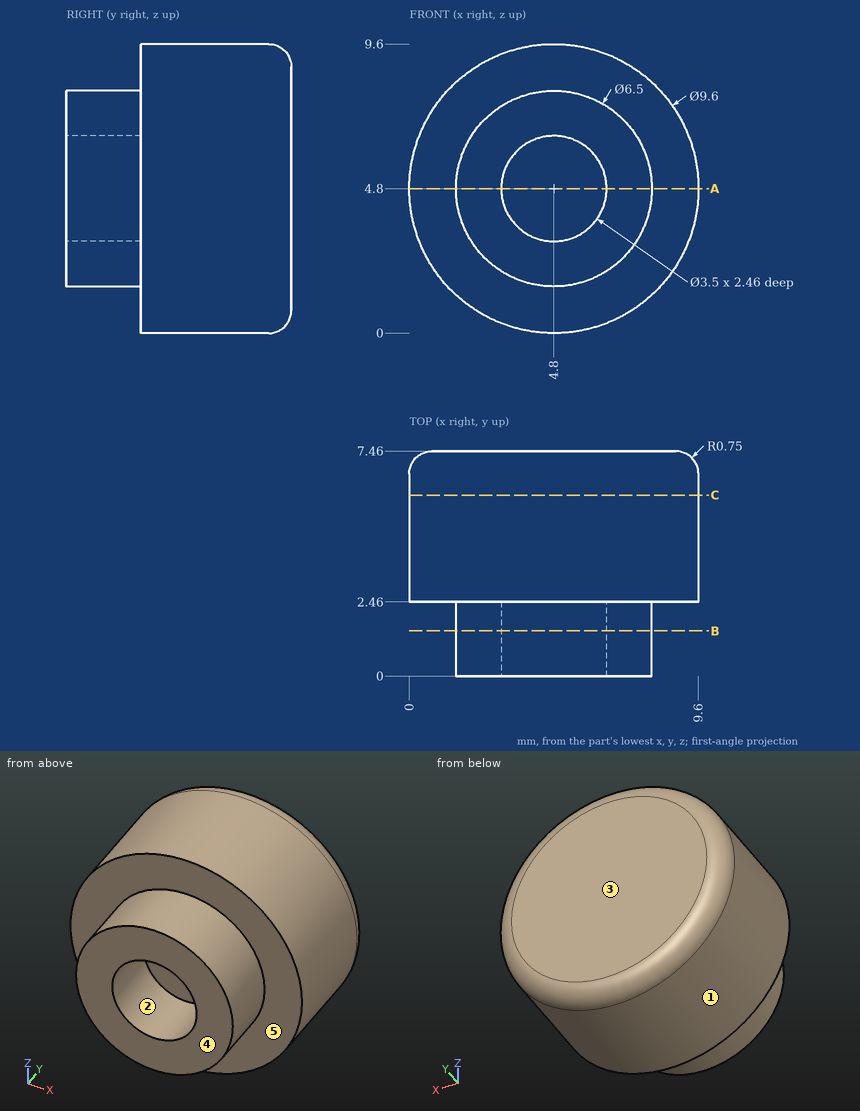
Geometry: see drawing. Coordinates: mm, zero at the bounding-box minimum. A direction names the side the tool comes from. Coordinates: 2 decimals unless noted, no trailing zeros. Loops run counter-clockwise (first coordinate to the right, second up) from the corner with the lowest first, then second, coordinate; pieces in that order, holes last.
(1) Section C-C on y = 6. Return the cut outline in (x, z).
(2) Section A-A on z = 4.8. Return the cut outline in (x, y).
(3) Material intervals for probe 1 along Z at (x, y) = (4.8, 1.4); probe 2 along Y at (x, z) = (1.5, 6.75); probe 3 along X at (y, z) = (1.25, 6.25), sorted ascending.
(4) Set-up query: the marked faces 4 and 5. Return all of +Z, -Z, +X, -X, +Y, -Y with unobstructed straight access to the full face (end or side cutting, diameter ignored); none if empty.
(5) First-contact query: pin 1 Ø4 at (x, y) = (7.5, 6) entering from -Z; pin 2 Ø1.5 at (y, z) = (3, 7) entering from -X; pin 3 Ø5 at (x, z) = (4.5, 4.5) entering from -Y; pin 4 Ø2 at (x, y) = (7, 2.5) entering from +Z. Flat tips, straight axial feed; report the tip coordinate or a pass-through.
(6) Pull-direction query (X, two-part tool) for the marked faces 1, 2 and 3; classes: released by +X, released by -X, zero draft, split by the parting line, or undercut.
(7) Section B-B on y = 1.5. Return the cut outline in (x, z), then the cut area to 3 significant figures.
Data:
1. outline: circle Ø9.6 at (4.8, 4.8)
2. outline: (0, 2.46) - (1.55, 2.46) - (1.55, 0) - (3.05, 0) - (3.05, 2.46) - (6.55, 2.46) - (6.55, 0) - (8.05, 0) - (8.05, 2.46) - (9.6, 2.46) - (9.6, 6.71) arc R0.75 ccw to (8.85, 7.46) - (0.75, 7.46) arc R0.75 ccw to (0, 6.71) - close
3. probe 1: z = 1.55 to 3.05, 6.55 to 8.05
3. probe 2: y = 2.46 to 7.46
3. probe 3: x = 1.89 to 3.82, 5.78 to 7.71
4. face 4: +Z, -Z, +X, -X, -Y
4. face 5: -Y
5. pin 1: stops at z = 0.05
5. pin 2: stops at x = 0.22
5. pin 3: stops at y = 0
5. pin 4: stops at z = 9.45
6. face 1: split by the parting line
6. face 2: undercut
6. face 3: zero draft
7. outline: circle Ø6.5 at (4.8, 4.8); hole circle Ø3.5 at (4.8, 4.8)
7. area: 23.6 mm2
